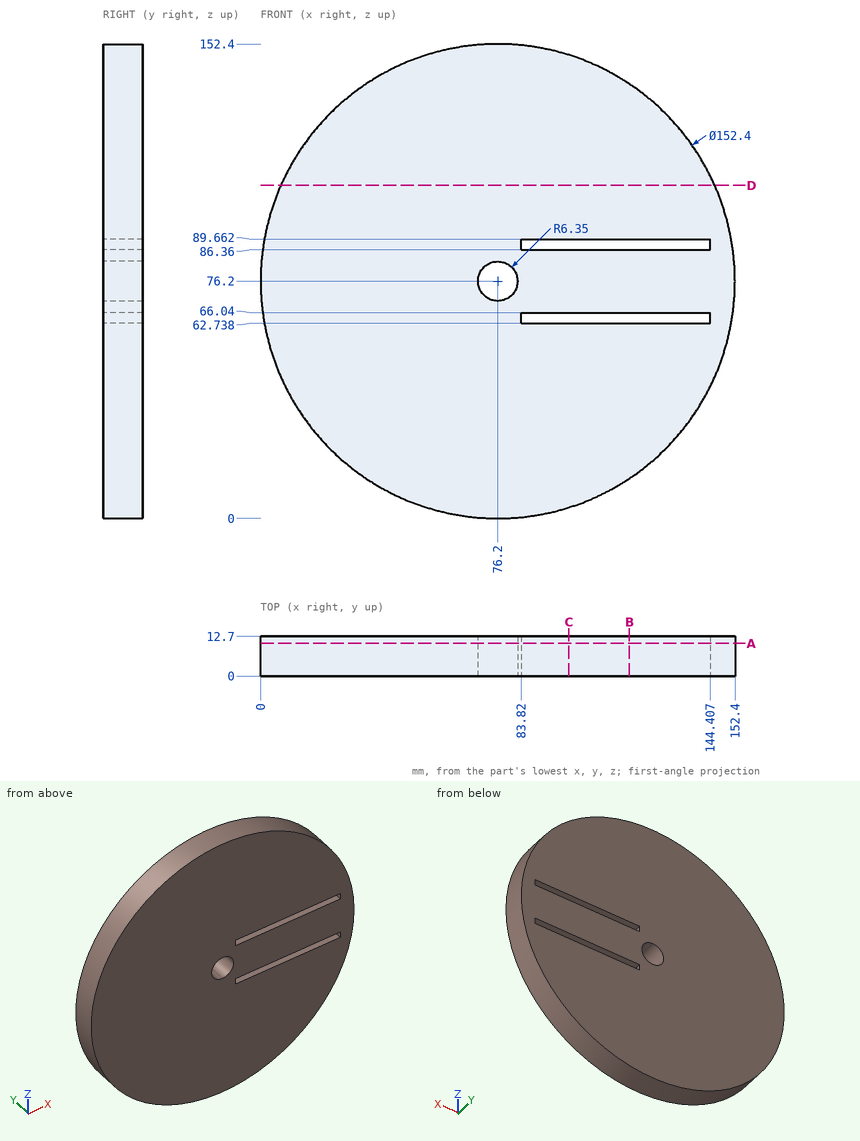
Design review of the part shown in the three views and the two pictorial views. Dimensions are in mm from the part's minimum x, y and z. Coordinates: 2 decimals unless noted, no trailing zeros. Write each loop counter-clockwise with the first axis right and the second up, starting at its lowest first coordinate (ties: lowest second). Pieces come first, ordered by that corner, then holes.
(1) Wall thickness on probe 1 along Z at (x, y) = (84, 11.5); probe 2 along Z at (x, y) = (88, 1); probe 3 along X at (y, z) = (8.5, 88): over which ranges is each line inside the solid? List them lowest first.
(2) Add section D-D on z = 107. Give the boundary of the cut face in (x, y), then the cut area to 3 significant figures.
(3) Add section B-B on x = 118.5. Give the boundary of the cut face in (y, z).
(4) For pin 1 Ø1 at (x, z) = (106, 106) entering from -Y; pin 2 Ø4 at (x, y) = (117.5, 9) entering from -Z; pin 3 Ø2.5 at (y, z) = (4.5, 64) entering from +X; pin 4 Ø5 at (x, y) = (96.5, 7.5) entering from -Z, all flat-tipped, find the tip position at first contact; note any pin that passes through.
(5) Add section C-C on x = 99. Give the boundary of the cut face in (y, z), then the cut area to 3 significant figures.
(6) Add section A-A on y = 10.5. Give the boundary of the cut face in (x, z).
Answer sheet:
1. probe 1: z = 0.4 to 62.74, 66.04 to 86.36, 89.66 to 152
1. probe 2: z = 0.92 to 62.74, 66.04 to 86.36, 89.66 to 151.48
1. probe 3: x = 0.92 to 83.82, 144.41 to 151.48
2. outline: (6.5, 0) - (145.9, 0) - (145.9, 12.7) - (6.5, 12.7) - close
2. area: 1,770 mm2
3. outline: (0, 12.82) - (12.7, 12.82) - (12.7, 62.74) - (0, 62.74) - close; (0, 66.04) - (12.7, 66.04) - (12.7, 86.36) - (0, 86.36) - close; (0, 89.66) - (12.7, 89.66) - (12.7, 139.58) - (0, 139.58) - close
4. pin 1: stops at y = 0
4. pin 2: stops at z = 10.92
4. pin 3: stops at x = 151.61
4. pin 4: stops at z = 2.11
5. outline: (0, 3.49) - (12.7, 3.49) - (12.7, 62.74) - (0, 62.74) - close; (0, 66.04) - (12.7, 66.04) - (12.7, 86.36) - (0, 86.36) - close; (0, 89.66) - (12.7, 89.66) - (12.7, 148.91) - (0, 148.91) - close
5. area: 1,760 mm2
6. outline: circle Ø152.4 at (76.2, 76.2); hole circle Ø12.7 at (76.2, 76.2); hole (83.82, 62.74) - (144.41, 62.74) - (144.41, 66.04) - (83.82, 66.04) - close; hole (83.82, 86.36) - (144.41, 86.36) - (144.41, 89.66) - (83.82, 89.66) - close
